For this review, take the finished solid that the model builds, in its own axes (mm). A direction names the side the tool comes from. Coordinates: 2 decimals unless noted, no trailing zeros. Loops run counter-clockwise (first coordinate to the right, second up) from the corner with the lowest first, then second, coordinate; pieces in that order, holes last. Notation, with made-up numbers: (-1, 68) - (51, 68) arc R31 ccw to (51, 94) - close; hole circle Ø2 at (71.5, -34). An arc over 180 degrees is marked (long way). Answer as a JSON object with one key per item and string values. Group by question number.
Item 1: To check wall thickness, follow line 1 (Z direction, x = 5, y = 7.75); line 2 (X direction, y = 8, z = -0.8); line 3 (X direction, y = 5.75, z = -1.15). State the ranges of each line that lie inside material, in increasing order.
Item 2: Clearance check with flat-ended pins moving along their axes: pin 1 (0.8 mm diameter, centred on x = 6.5, y = 0, fed in from -Z); pin 2 (1.5 mm diameter, centred on x = 3.5, z = -2, fed in from +Y). State where each tip first meets the part, or that it passes through.
Item 3: We need section A-A (y = 5). Give the boundary of the cut face in (x, z) (3 decimals), then the cut area to 3 significant figures.
Item 4: We need section C-C (z = -2.65). Give the boundary of the cut face in (x, y).
Item 5: Tool access review of faces 4 (the flat face through (4, 5, -2.99)), 5 (the flat face through (4, 5, -1.92)): name each direction out of +Z, -Z, +X, -X, +Y, -Y from which nothing blocks a thin tool from reaching the whole face with its end or side.
Item 6: We need section B-B (x = 1.75). Give the boundary of the cut face in (y, z).
Item 7: We need section D-D (y = 1.75). Give the boundary of the cut face in (x, z), then the cut area to 3 significant figures.
Item 8: Mouldability with a two-part tool opening along Z and no side actions: class faces 1 (the cylindrical face through (0.23, 0.35, -2.6)), 2 (the flat face through (8.65, 6, -1)), 3 (the cylindrical face through (8.707, 4.788, -0.389)) as released by +Z, released by -Z, zero draft, split by the parting line, or undercut.
from build123d import *

# Parameters (mm, degrees)
EXTRUDE_1_DEPTH     = 9.3
EXTRUDE_2_DEPTH     = 0.15
EXTRUDE_START       = -0.15
EXTRUDE_3_DEPTH     = 0.15
EXTRUDE_4_DEPTH     = 2
CUT_EXTRUDE_1_DEPTH = 0.7
FILLET_1_R          = 0.3
EXTRUDE_5_DEPTH     = 0.15
CUT_EXTRUDE_2_DEPTH = 0.15
EXTRUDE_6_DEPTH     = 6.9
FILLET_2_R          = 0.2


with BuildPart() as part:
    # 草图1 → 凸台-拉伸1 (new body)
    with BuildSketch(Plane(origin=(0, 0, 0), x_dir=(1, 0, 0), z_dir=(0, 1, 0))):
        with BuildLine():
            Line((0.8, -0.15), (7.85, -0.15))
            ThreePointArc((7.85, -0.15), (8.521751442, 0.128248558), (8.8, 0.8))
            Line((8.8, 0.8), (8.8, 2.04))
            ThreePointArc((8.8, 2.04), (8.521751442, 2.711751442), (7.85, 2.99))
            Line((7.85, 2.99), (0.8, 2.99))
            ThreePointArc((0.8, 2.99), (0.128248558, 2.711751442), (-0.15, 2.04))
            Line((-0.15, 2.04), (-0.15, 0.8))
            ThreePointArc((-0.15, 0.8), (0.128248558, 0.128248558), (0.8, -0.15))
        make_face()
        with BuildLine():
            Line((0.8, 0), (7.85, 0))
            ThreePointArc((7.85, 0), (8.415685425, 0.234314575), (8.65, 0.8))
            Line((8.65, 0.8), (8.65, 2.04))
            ThreePointArc((8.65, 2.04), (8.415685425, 2.605685425), (7.85, 2.84))
            Line((7.85, 2.84), (0.8, 2.84))
            ThreePointArc((0.8, 2.84), (0.234314575, 2.605685425), (0, 2.04))
            Line((0, 2.04), (0, 0.8))
            ThreePointArc((0, 0.8), (0.234314575, 0.234314575), (0.8, 0))
        make_face(mode=Mode.SUBTRACT)
    extrude(amount=EXTRUDE_1_DEPTH)

    # 草图3 → 凸台-拉伸2 (add)
    with BuildSketch(Plane.ZY.offset(0.15)):
        with BuildLine():
            Line((-2.04, 0), (-0.8, 0))
            Line((-0.8, 0), (-0.683566262, -0.646854101))
            ThreePointArc((-0.683566262, -0.646854101), (-0.748665041, -0.892426908), (-0.978821259, -1))
            Line((-0.978821259, -1), (-1.12, -1))
            ThreePointArc((-1.12, -1), (-1.226066017, -0.956066017), (-1.27, -0.85))
            Line((-1.27, -0.85), (-1.27, -0.45))
            ThreePointArc((-1.27, -0.45), (-1.313933983, -0.343933983), (-1.42, -0.3))
            ThreePointArc((-1.42, -0.3), (-1.526066017, -0.343933983), (-1.57, -0.45))
            Line((-1.57, -0.45), (-1.57, -0.85))
            ThreePointArc((-1.57, -0.85), (-1.613933983, -0.956066017), (-1.72, -1))
            Line((-1.72, -1), (-1.861178741, -1))
            ThreePointArc((-1.861178741, -1), (-2.091334959, -0.892426908), (-2.156433738, -0.646854101))
            Line((-2.156433738, -0.646854101), (-2.04, 0))
        make_face()
    extrude(amount=-EXTRUDE_2_DEPTH)

    # 草图4 → 凸台-拉伸3 (add)
    with BuildSketch(Plane(origin=(8.8, 0, 0), x_dir=(0, 0, -1), z_dir=(1, 0, 0)).offset(EXTRUDE_START)):
        with BuildLine():
            Line((0.8, 0), (2.04, 0))
            Line((2.04, 0), (2.156433738, -0.646854101))
            ThreePointArc((2.156433738, -0.646854101), (2.091334959, -0.892426908), (1.861178741, -1))
            Line((1.861178741, -1), (1.72, -1))
            ThreePointArc((1.72, -1), (1.613933983, -0.956066017), (1.57, -0.85))
            Line((1.57, -0.85), (1.57, -0.45))
            ThreePointArc((1.57, -0.45), (1.42, -0.3), (1.27, -0.45))
            Line((1.27, -0.45), (1.27, -0.85))
            ThreePointArc((1.27, -0.85), (1.226066017, -0.956066017), (1.12, -1))
            Line((1.12, -1), (0.978821259, -1))
            ThreePointArc((0.978821259, -1), (0.748665041, -0.892426908), (0.683566262, -0.646854101))
            Line((0.683566262, -0.646854101), (0.8, 0))
        make_face()
    extrude(amount=EXTRUDE_3_DEPTH)

    # 草图5 → 凸台-拉伸4 (add)
    with BuildSketch(Plane.XZ):
        with BuildLine():
            Line((0.8, -2.99), (7.85, -2.99))
            ThreePointArc((7.85, -2.99), (8.521751442, -2.711751442), (8.8, -2.04))
            Line((8.8, -2.04), (8.8, -0.8))
            ThreePointArc((8.8, -0.8), (8.521751442, -0.128248558), (7.85, 0.15))
            Line((7.85, 0.15), (0.8, 0.15))
            ThreePointArc((0.8, 0.15), (0.128248558, -0.128248558), (-0.15, -0.8))
            Line((-0.15, -0.8), (-0.15, -2.04))
            ThreePointArc((-0.15, -2.04), (0.128248558, -2.711751442), (0.8, -2.99))
        make_face()
    extrude(amount=-EXTRUDE_4_DEPTH)

    # 草图6 → 切除-拉伸1 (cut)
    with BuildSketch(Plane.XZ):
        with BuildLine():
            Line((0.8, 0.15), (7.85, 0.15))
            ThreePointArc((7.85, 0.15), (8.521751442, -0.128248558), (8.8, -0.8))
            Line((8.8, -0.8), (8.65, -0.8))
            ThreePointArc((8.65, -0.8), (8.415685425, -0.234314575), (7.85, 0))
            Line((7.85, 0), (0.8, 0))
            ThreePointArc((0.8, 0), (0.234314575, -0.234314575), (0, -0.8))
            Line((0, -0.8), (-0.15, -0.8))
            ThreePointArc((-0.15, -0.8), (0.128248558, -0.128248558), (0.8, 0.15))
        make_face()
        with BuildLine():
            Line((7.85, -2.99), (0.8, -2.99))
            ThreePointArc((0.8, -2.99), (0.128248558, -2.711751442), (-0.15, -2.04))
            Line((-0.15, -2.04), (0, -2.04))
            ThreePointArc((0, -2.04), (0.234314575, -2.605685425), (0.8, -2.84))
            Line((0.8, -2.84), (7.85, -2.84))
            ThreePointArc((7.85, -2.84), (8.415685425, -2.605685425), (8.65, -2.04))
            Line((8.65, -2.04), (8.8, -2.04))
            ThreePointArc((8.8, -2.04), (8.521751442, -2.711751442), (7.85, -2.99))
        make_face()
    extrude(amount=-CUT_EXTRUDE_1_DEPTH, mode=Mode.SUBTRACT)

    # 圆角1
    fillet_1_edges = [part.edges().sort_by_distance(p)[0] for p in [
        (8.725, 0.7, -0.8),
        (-0.075, 0.7, -0.8),
        (-0.075, 0.7, -2.04),
        (8.725, 0.7, -2.04),
    ]]
    fillet(fillet_1_edges, radius=FILLET_1_R)

    # 草图7 → 凸台-拉伸5 (add)
    with BuildSketch(Plane(origin=(0, 0, -2.99), x_dir=(-1, 0, 0), z_dir=(0, 0, -1))):
        with BuildLine():
            Line((-3.225, 0.7), (-5.425, 0.7))
            ThreePointArc((-5.425, 0.7), (-5.071446609, 0.553553391), (-4.925, 0.2))
            Line((-4.925, 0.2), (-4.925, -0.9))
            ThreePointArc((-4.925, -0.9), (-4.837132034, -1.112132034), (-4.625, -1.2))
            Line((-4.625, -1.2), (-4.325, -1.2))
            Line((-4.325, -1.2), (-4.025, -1.2))
            ThreePointArc((-4.025, -1.2), (-3.812867966, -1.112132034), (-3.725, -0.9))
            Line((-3.725, -0.9), (-3.725, 0.2))
            ThreePointArc((-3.725, 0.2), (-3.578553391, 0.553553391), (-3.225, 0.7))
        make_face()
    extrude(amount=-EXTRUDE_5_DEPTH)

    # 草图8 → 切除-拉伸2 (cut)
    with BuildSketch(Plane(origin=(0, 0, -2.99), x_dir=(-1, 0, 0), z_dir=(0, 0, -1))):
        with BuildLine():
            Line((-4.325, -0.9), (-4.125, -0.9))
            ThreePointArc((-4.125, -0.9), (-4.054289322, -0.870710678), (-4.025, -0.8))
            Line((-4.025, -0.8), (-4.025, -0.4))
            ThreePointArc((-4.025, -0.4), (-4.054289322, -0.329289322), (-4.125, -0.3))
            Line((-4.125, -0.3), (-4.525, -0.3))
            ThreePointArc((-4.525, -0.3), (-4.595710678, -0.329289322), (-4.625, -0.4))
            Line((-4.625, -0.4), (-4.625, -0.8))
            ThreePointArc((-4.625, -0.8), (-4.595710678, -0.870710678), (-4.525, -0.9))
            Line((-4.525, -0.9), (-4.325, -0.9))
        make_face()
    extrude(amount=-CUT_EXTRUDE_2_DEPTH, mode=Mode.SUBTRACT)

    # 草图9 → 凸台-拉伸6 (add)
    with BuildSketch(Plane(origin=(0, 2, 0), x_dir=(1, 0, 0), z_dir=(0, 1, 0))):
        with BuildLine():
            Line((1.325, 1.42), (1.325, 1.62))
            ThreePointArc((1.325, 1.62), (1.412867966, 1.832132034), (1.625, 1.92))
            Line((1.625, 1.92), (7.025, 1.92))
            ThreePointArc((7.025, 1.92), (7.237132034, 1.832132034), (7.325, 1.62))
            Line((7.325, 1.62), (7.325, 1.22))
            ThreePointArc((7.325, 1.22), (7.237132034, 1.007867966), (7.025, 0.92))
            Line((7.025, 0.92), (1.625, 0.92))
            ThreePointArc((1.625, 0.92), (1.412867966, 1.007867966), (1.325, 1.22))
            Line((1.325, 1.22), (1.325, 1.42))
        make_face()
    extrude(amount=EXTRUDE_6_DEPTH)

    # 圆角2
    fillet_2_edges = [part.edges().sort_by_distance(p)[0] for p in [
        (7.325, 8.9, -1.42),
        (7.237132034, 8.9, -1.007867966),
        (4.325, 8.9, -0.92),
        (1.412867966, 8.9, -1.007867966),
        (1.325, 8.9, -1.42),
        (1.412867966, 8.9, -1.832132034),
        (4.325, 8.9, -1.92),
        (7.237132034, 8.9, -1.832132034),
    ]]
    fillet(fillet_2_edges, radius=FILLET_2_R)


solid = part.part
Check sheet entries:
{
 "1": {"line 1": "z = -2.99 to -2.84, -1.92 to -0.92, 0 to 0.15", "line 2": "x = -0.15 to 0, 8.65 to 8.8", "line 3": "x = -0.15 to 0, 1.33 to 7.32, 8.65 to 8.8"},
 "2": {"pin 1": "stops at z = -2.84", "pin 2": "stops at y = 8.9"},
 "3": {"outline": "(-0.15, -2.04) arc R0.95 ccw to (0.8, -2.99) - (7.85, -2.99) arc R0.95 ccw to (8.8, -2.04) - (8.8, -0.8) arc R0.95 ccw to (7.85, 0.15) - (0.8, 0.15) arc R0.95 ccw to (-0.15, -0.8) - close; (1.325, -1.62) arc R0.3 ccw to (1.625, -1.92) - (7.025, -1.92) arc R0.3 ccw to (7.325, -1.62) - (7.325, -1.22) arc R0.3 ccw to (7.025, -0.92) - (1.625, -0.92) arc R0.3 ccw to (1.325, -1.22) - close; hole (0, -2.04) arc R0.8 ccw to (0.8, -2.84) - (7.85, -2.84) arc R0.8 ccw to (8.65, -2.04) - (8.65, -0.8) arc R0.8 ccw to (7.85, 0) - (0.8, 0) arc R0.8 ccw to (0, -0.8) - close", "area": "9.23 mm2"},
 "4": {"outline": "(0.07, 0.7) - (0.28, 0.7) - (0.28, 0) - (8.37, 0) - (8.37, 0.7) - (8.58, 0.7) - (8.58, 9.3) - (8.37, 9.3) - (8.37, 2) - (0.28, 2) - (0.28, 9.3) - (0.07, 9.3) - close"},
 "5": {"face 4": "-Z, +X, -X, +Y, -Y", "face 5": "+Y"},
 "6": {"outline": "(0, -2.84) - (0.7, -2.84) - (0.7, -2.99) - (9.3, -2.99) - (9.3, -2.84) - (2, -2.84) - (2, -1.92) - (8.7, -1.92) arc R0.2 ccw to (8.9, -1.72) - (8.9, -1.12) arc R0.2 ccw to (8.7, -0.92) - (2, -0.92) - (2, 0) - (9.3, 0) - (9.3, 0.15) - (0.7, 0.15) - (0.7, 0) - (0, 0) - close"},
 "7": {"outline": "(-0.15, -2.04) arc R0.95 ccw to (0.8, -2.99) - (7.85, -2.99) arc R0.95 ccw to (8.8, -2.04) - (8.8, -0.8) arc R0.95 ccw to (7.85, 0.15) - (0.8, 0.15) arc R0.95 ccw to (-0.15, -0.8) - close", "area": "27.3 mm2"},
 "8": {"face 1": "released by -Z", "face 2": "undercut", "face 3": "released by +Z"}
}
